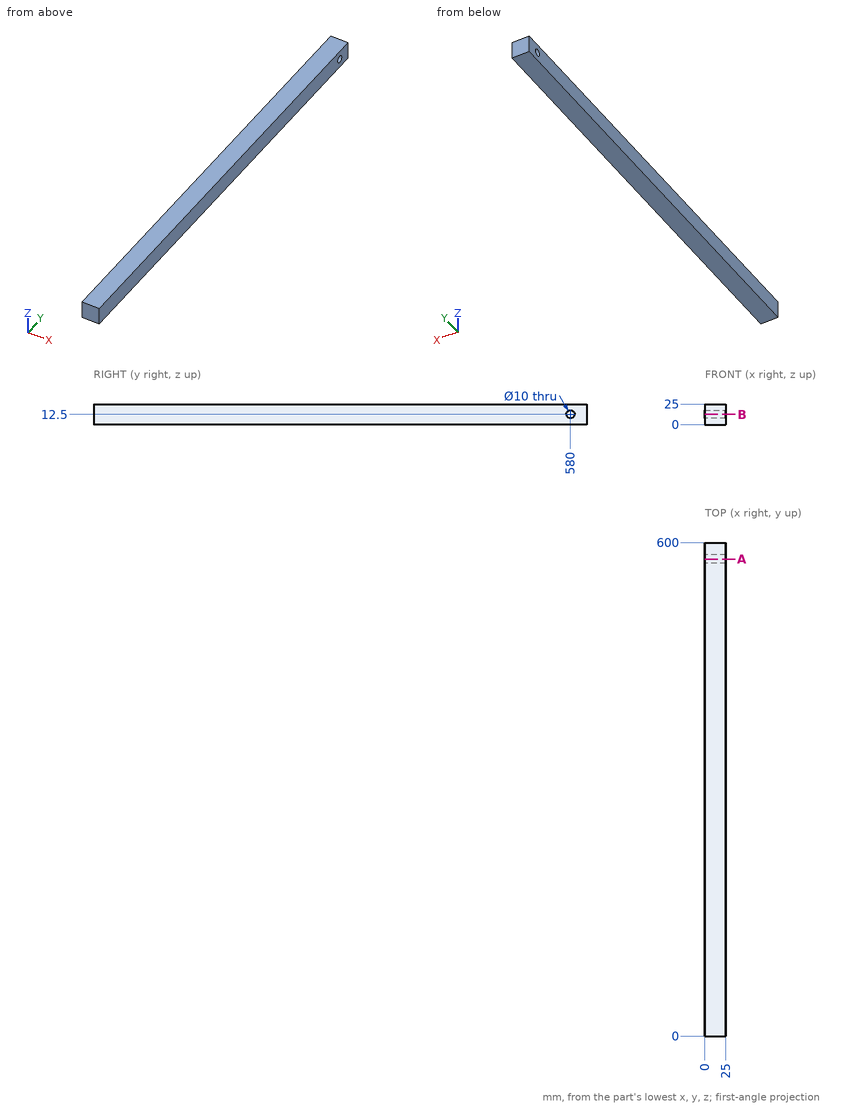
Input: dimensioned drawing with shaded views. Units: mm. Origin: part minimum x, y, z. Give positions to 0.01 mm unless a question says otherwise; leave off trailing zeros. Write each loop counter-clockwise with the first axis right and the second up, starting at its lowest first coordinate (ties: lowest second). Pieces come first, ordered by that corner, then holes. Notation, with made-up numbers: M -22,61 L -1,61 A25 ccw -1,100 Z; hole C -6,-28 d10. An arc over 180 degrees is marked long. Return JSON: item names as keys, results as strings. Group by question number.
1) Pin query (flat end, axial travel): P1, Ø11.5, axis at y = 580, z = 12.5, coming from the -X side. Return the tip coordinate at first contact, or that it passes through.
2) Cut plane B-B, the plane z = 12.5. Output: boundary loops of the cut face in (x, y), plus the area to 4 significant figures.
3) Cut plane A-A, the plane y = 580. Output: boundary loops of the cut face in (x, z), plus the area to 3 significant figures.
4) Material intervals for line 1 along Y through (x, z) = (15.75, 12.5); line 2 along Y through (x, z) = (10.75, 9), sorted ascending. Write a range as [from, to].
Recorded:
{
 "1": {"P1": "stops at x = 0"},
 "2": {"outline": "M 0,0 L 25,0 L 25,575 L 0,575 Z; M 0,585 L 25,585 L 25,600 L 0,600 Z", "area": "14,750 mm²"},
 "3": {"outline": "M 0,0 L 25,0 L 25,7.5 L 0,7.5 Z; M 0,17.5 L 25,17.5 L 25,25 L 0,25 Z", "area": "375 mm²"},
 "4": {"line 1": "y = [0, 575], [585, 600]", "line 2": "y = [0, 576.43], [583.57, 600]"}
}
